Work out the finished part from the listing and answer in its coordinate system (mm). A direction names the side the tool comes from. Give positions to 0.01 mm unless a question says otherwise; leave off trailing zeros. Loops run counter-clockwise (first coordinate to the right, second up) from the corner with the lowest first, then second, coordinate; pieces in that order, holes last.
```python
from build123d import *

# Parameters (mm, degrees)
F0_W     = 40
F0_H     = 22
F0_W_2   = 34
F0_H_2   = 4.5532393306
F1_DEPTH = 5
F2_DEPTH = 48


with BuildPart() as f1:
    # F0 (on Top) → F1 (new body)
    with BuildSketch(Plane.XY):
        Rectangle(F0_W, F0_H)
        Polygon((17, -3.9467606694), (17, -8.5), (-17, -8.5), (-17, -3.9467606694), (-17, 3.9467606694), (-17, 8.5), (17, 8.5), (17, 3.9467606694), align=None, mode=Mode.SUBTRACT)
        with Locations((0, -6.2233803347)):
            Rectangle(F0_W_2, F0_H_2)
        with Locations((0, 6.2233803347)):
            Rectangle(F0_W_2, F0_H_2)
    extrude(amount=F1_DEPTH)

    # F0 (on Top) → F2 (join)
    with BuildSketch(Plane.XY):
        Rectangle(F0_W, F0_H)
        Polygon((17, -3.9467606694), (17, -8.5), (-17, -8.5), (-17, -3.9467606694), (-17, 3.9467606694), (-17, 8.5), (17, 8.5), (17, 3.9467606694), align=None, mode=Mode.SUBTRACT)
    extrude(amount=F2_DEPTH)


solid = f1.part
```
Q1. Section B-B on x = -11.5 is taken. Give the vertices of the cut face in (y, z), plus the area to 3 significant figures.
Q2. Section D-D on y = 6.5 is taken. Give the vertices of the cut face in (x, z).
Q3. Consider line 1 along X through (y, z) = (-0.75, 10); line 2 along Y through (x, z) = (-3, 23); line 3 along Y through (x, z) = (-6, 4). Determine where each line is inside the solid, lowest interval first.
Q4. Determine the mould class of faces 4 (the face through (0, -11, 24)), 5 (the face through (20, 0, 24)), 6 (the face through (-20, 0, 24)), 7 (the face through (0, -8.5, 26)) for opening direction X: +X half, -X half, draft (parallel to the pull), parting line (faces both ways), or undercut.
Q5. Section C-C on z = 45.5 is taken. Give the vertices of the cut face in (x, y), plus the area to 3 significant figures.
Q6. Section A-A on y = 2.25 is taken. Give the vertices of the cut face in (x, z).
Q7. Which of the six approach directions +Z, -Z, +X, -X, +Y, -Y give full straight-line access (tool end or side, diameter ignored) to faces 1 (the face through (0, 11, 24)), 2 (the face through (0, 3.947, 2)), 3 (the face through (0, 8.5, 26))?
Check result:
1. outline: (-11, 0) - (-3.95, 0) - (-3.95, 5) - (-8.5, 5) - (-8.5, 48) - (-11, 48) - close; (3.95, 0) - (11, 0) - (11, 48) - (8.5, 48) - (8.5, 5) - (3.95, 5) - close
1. area: 286 mm2
2. outline: (-20, 0) - (20, 0) - (20, 48) - (17, 48) - (17, 5) - (-17, 5) - (-17, 48) - (-20, 48) - close
3. line 1: x = -20 to -17, 17 to 20
3. line 2: y = -11 to -8.5, 8.5 to 11
3. line 3: y = -11 to -3.95, 3.95 to 11
4. face 4: draft
4. face 5: +X half
4. face 6: -X half
4. face 7: undercut
5. outline: (-20, -11) - (20, -11) - (20, 11) - (-20, 11) - close; hole (-17, -8.5) - (17, -8.5) - (17, 8.5) - (-17, 8.5) - close
5. area: 302 mm2
6. outline: (-20, 0) - (-17, 0) - (-17, 48) - (-20, 48) - close; (17, 0) - (20, 0) - (20, 48) - (17, 48) - close
7. face 1: +Z, -Z, +X, -X, +Y
7. face 2: +Z, -Z
7. face 3: +Z
